Read the model definition and answer for the solid it produces. Units are mm, in the model's axes. Face numbers are marked on the shaded views. A direction names the side the tool comes from. Round coordinates to 2 decimals unless told otherwise and drop trailing zeros. Write each loop counter-clockwise with the first axis right and the second up, starting at its lowest first coordinate (ties: lowest second). Pieces come first, ordered by that corner, then holes. Notation, with made-up numbers: (-30, 40.25) -> (-7, 40.25) arc R8 ccw to (-7, 46.25) -> close; hole circle Ø10 at (61, 18). An arc over 180 degrees is marked (long way). Return JSON: item names as keys, results as strings. Group by question number.
(1) A cutting plane is placed at A-A on z = -1. State how many separate pieces and enclosed holes the cut face has, then the cut area to 3 significant figures.
(2) For the marked faces 1, 2, 3 and 4, determine the directions among +Z, -Z, +X, -X, +Y, -Y from which every point of the face is accessible in a straight line to the end or side of a thin tool.
(3) A cutting plane is placed at D-D on x = 18.75. Give the vertices of the cut face in (y, z), then the cut area to 3 significant figures.
(4) The mould has two halves that part along X. Classify the marked faces 5, 6 and 7: released by +X, released by -X, zero draft, split by the parting line, or undercut.
(5) A cutting plane is placed at C-C on z = -8.5. Give the vertices of the cut face in (x, y).
(6) Straight lines are drawn through the part: line 1 (Z direction, x = 11.5, y = 9.5); line 2 (Y direction, x = 7.75, z = 1); line 3 (Y direction, x = 11, z = -6.5). For each, find the intervals that lie inside material, in ascending order.
(7) Given pin 1 (3 mm diameter, centred on x = 8.5, y = 4, fed in from -Z); pin 2 (1 mm diameter, centred on x = 11.5, y = 10, fed in from -Z); pin 3 (2 mm diameter, centred on x = 15, z = 0.5, fed in from +Y); pin 4 (1.5 mm diameter, centred on y = 6.5, z = -6.5, fed in from +X), each flat-ended and moving along its own axis, determine where each tip first touches the part or whether it passes through.
```python
from build123d import *

# Parameters (mm, degrees)
BOSS_EXTRUDE1_DEPTH   = 8
BOSS_EXTRUDE1_2_DEPTH = 8
BOSS_EXTRUDE1_3_DEPTH = 8
BOSS_EXTRUDE1_4_DEPTH = 8
BOSS_EXTRUDE1_5_DEPTH = 8
BOSS_EXTRUDE1_6_DEPTH = 8
BOSS_EXTRUDE1_7_DEPTH = 8
BASE_W                = 23
BASE_H                = 3
BOSS_EXTRUDE2_DEPTH   = 8
SKETCH1_W             = 5
SKETCH1_H             = 7
BOSS_EXTRUDE3_DEPTH   = 2
SKETCH2_W             = 2
SKETCH2_H             = 3
BOSS_EXTRUDE4_DEPTH   = 14


with BuildPart() as part:
    # Gears-1 → Boss-Extrude1 (new body)
    with BuildSketch(Plane(origin=(0, 0, 0), x_dir=(1, 0, 0), z_dir=(0, 1, 0))):
        with BuildLine():
            Line((-0.500594601, 0), (0.709644096, 3.775809937))
            ThreePointArc((0.709644096, 3.775809937), (0.980506814, 3.882987586), (1.251369531, 3.775809937))
            Line((1.251369531, 3.775809937), (2.579049224, 0))
            Line((2.579049224, 0), (-0.500594601, 0))
        make_face()
    extrude(amount=BOSS_EXTRUDE1_DEPTH)



with BuildPart() as body_2:
    # Gears-1 → Boss-Extrude1 2 (new body)
    with BuildSketch(Plane(origin=(0, 0, 0), x_dir=(1, 0, 0), z_dir=(0, 1, 0))):
        with BuildLine():
            Line((2.599405399, 0), (5.679049224, 0))
            Line((5.679049224, 0), (4.351369531, 3.775809937))
            ThreePointArc((4.351369531, 3.775809937), (4.080506814, 3.882987586), (3.809644096, 3.775809937))
            Line((3.809644096, 3.775809937), (2.599405399, 0))
        make_face()
    extrude(amount=BOSS_EXTRUDE1_2_DEPTH)


with BuildPart() as body_3:
    # Gears-1 → Boss-Extrude1 3 (new body)
    with BuildSketch(Plane(origin=(0, 0, 0), x_dir=(1, 0, 0), z_dir=(0, 1, 0))):
        with BuildLine():
            Line((5.699405399, 0), (8.779049224, 0))
            Line((8.779049224, 0), (7.451369531, 3.775809937))
            ThreePointArc((7.451369531, 3.775809937), (7.180506814, 3.882987586), (6.909644096, 3.775809937))
            Line((6.909644096, 3.775809937), (5.699405399, 0))
        make_face()
    extrude(amount=BOSS_EXTRUDE1_3_DEPTH)


with BuildPart() as body_4:
    # Gears-1 → Boss-Extrude1 4 (new body)
    with BuildSketch(Plane(origin=(0, 0, 0), x_dir=(1, 0, 0), z_dir=(0, 1, 0))):
        with BuildLine():
            Line((8.799405399, 0), (11.879049224, 0))
            Line((11.879049224, 0), (10.551369531, 3.775809937))
            ThreePointArc((10.551369531, 3.775809937), (10.280506814, 3.882987586), (10.009644096, 3.775809937))
            Line((10.009644096, 3.775809937), (8.799405399, 0))
        make_face()
    extrude(amount=BOSS_EXTRUDE1_4_DEPTH)


with BuildPart() as body_5:
    # Gears-1 → Boss-Extrude1 5 (new body)
    with BuildSketch(Plane(origin=(0, 0, 0), x_dir=(1, 0, 0), z_dir=(0, 1, 0))):
        with BuildLine():
            Line((11.899405399, 0), (14.979049224, 0))
            Line((14.979049224, 0), (13.651369531, 3.775809937))
            ThreePointArc((13.651369531, 3.775809937), (13.380506814, 3.882987586), (13.109644096, 3.775809937))
            Line((13.109644096, 3.775809937), (11.899405399, 0))
        make_face()
    extrude(amount=BOSS_EXTRUDE1_5_DEPTH)


with BuildPart() as body_6:
    # Gears-1 → Boss-Extrude1 6 (new body)
    with BuildSketch(Plane(origin=(0, 0, 0), x_dir=(1, 0, 0), z_dir=(0, 1, 0))):
        with BuildLine():
            Line((14.999405399, 0), (18.079049224, 0))
            Line((18.079049224, 0), (16.751369531, 3.775809937))
            ThreePointArc((16.751369531, 3.775809937), (16.480506814, 3.882987586), (16.209644096, 3.775809937))
            Line((16.209644096, 3.775809937), (14.999405399, 0))
        make_face()
    extrude(amount=BOSS_EXTRUDE1_6_DEPTH)


with BuildPart() as body_7:
    # Gears-1 → Boss-Extrude1 7 (new body)
    with BuildSketch(Plane(origin=(0, 0, 0), x_dir=(1, 0, 0), z_dir=(0, 1, 0))):
        with BuildLine():
            Line((18.099405399, 0), (21.179049224, 0))
            Line((21.179049224, 0), (19.851369531, 3.775809937))
            ThreePointArc((19.851369531, 3.775809937), (19.580506814, 3.882987586), (19.309644096, 3.775809937))
            Line((19.309644096, 3.775809937), (18.099405399, 0))
        make_face()
    extrude(amount=BOSS_EXTRUDE1_7_DEPTH)


with BuildPart() as part_1:
    add(part.part)

    add(body_2.part)  # Boss-Extrude2 merges body 2

    add(body_3.part)  # Boss-Extrude2 merges body 3

    add(body_4.part)  # Boss-Extrude2 merges body 4

    add(body_5.part)  # Boss-Extrude2 merges body 5

    add(body_6.part)  # Boss-Extrude2 merges body 6

    add(body_7.part)  # Boss-Extrude2 merges body 7
    # Base → Boss-Extrude2 (add)
    with BuildSketch(Plane(origin=(0, 0, 0), x_dir=(1, 0, 0), z_dir=(0, 1, 0))):
        with Locations((10.726532056, -1.5)):
            Rectangle(BASE_W, BASE_H)
    extrude(amount=BOSS_EXTRUDE2_DEPTH)

    # Sketch1 → Boss-Extrude3 (add)
    with BuildSketch(Plane(origin=(10, 0, 0), x_dir=(0, 0, -1), z_dir=(1, 0, 0))):
        with Locations((-0.5, 11.5)):
            Rectangle(SKETCH1_W, SKETCH1_H)
    extrude(amount=BOSS_EXTRUDE3_DEPTH)

    # Sketch2 → Boss-Extrude4 (add)
    with BuildSketch(Plane(origin=(0, 0, -2), x_dir=(-1, 0, 0), z_dir=(0, 0, -1))):
        with Locations((-11, 13.5)):
            Rectangle(SKETCH2_W, SKETCH2_H)
    extrude(amount=BOSS_EXTRUDE4_DEPTH)


solid = part_1.part
```
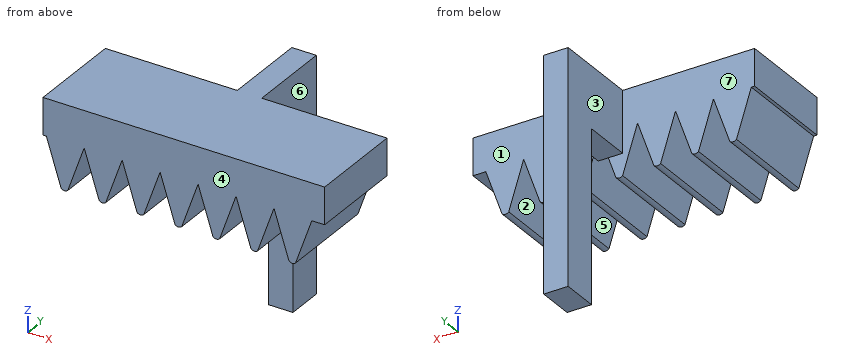
Checks:
{
 "1": {"separate pieces": "7", "enclosed holes": "0", "area": "149 mm^2"},
 "2": {"face 1": "+Z, -Z, +X, +Y", "face 2": "-Z, +Y, -Y", "face 3": "+Z, -Z, -X, +Y", "face 4": "+Z, -Z, +X, -X, -Y"},
 "3": {"outline": "(0, -2.03) -> (8, -2.03) -> (8, 3) -> (0, 3) -> close", "area": "40.2 mm^2"},
 "4": {"face 5": "undercut", "face 6": "released by +X", "face 7": "zero draft"},
 "5": {"outline": "(10, 12) -> (12, 12) -> (12, 15) -> (10, 15) -> close"},
 "6": {"line 1": "z = -2 to 3", "line 2": "y = 0 to 8", "line 3": "y = 12 to 15"},
 "7": {"pin 1": "stops at z = -3.88", "pin 2": "stops at z = -2", "pin 3": "stops at y = 8", "pin 4": "passes through"}
}
